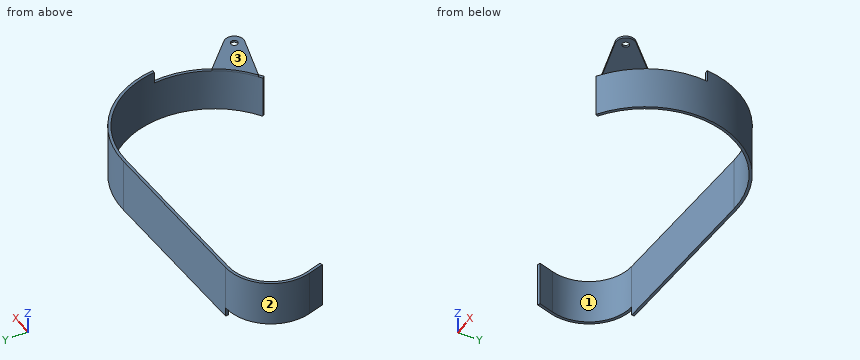
```python
from build123d import *

# Parameters (mm, degrees)
BASE_FLANGE1_DEPTH  = 52.5018
CUT_EXTRUDE1_DEPTH  = 8.89
CUT_EXTRUDE2_START  = -11.43
CUT_EXTRUDE2_DEPTH  = 11.43
SKETCH10_R          = 3.302
BOSS_EXTRUDE2_DEPTH = 2.032


# Sheet-metal steps are written as plain solids
with BuildPart() as part:
    # Sketch2 → Base-Flange1 (new body)
    with BuildSketch(Plane.XY):
        with BuildLine():
            Line((-203.2, 12.573), (-207.631458356, 27.163090613))
            ThreePointArc((-207.631458356, 27.163090613), (-201.190368302, 66.028990192), (-166.399327165, 84.512205491))
            Line((-166.399327165, 84.512205491), (-2.61152029, 89.301967603))
            ThreePointArc((-2.61152029, 89.301967603), (85.351357983, 26.397104888), (48.26, -75.184))
            Line((48.26, -75.184), (46.819332757, -72.939592084))
            ThreePointArc((46.819332757, -72.939592084), (82.803432048, 25.609093195), (-2.533560661, 86.636107274))
            Line((-2.533560661, 86.636107274), (-166.321367535, 81.846345161))
            ThreePointArc((-166.321367535, 81.846345161), (-199.024946204, 64.47212278), (-205.079570854, 27.938177176))
            Line((-205.079570854, 27.938177176), (-200.648112499, 13.348086563))
            Line((-200.648112499, 13.348086563), (-203.2, 12.573))
        make_face()
    extrude(amount=BASE_FLANGE1_DEPTH)

    # Sketch7 → Cut-Extrude1 (cut)
    with BuildSketch(Plane(origin=(0, 0, 0), x_dir=(-1, 0, 0), z_dir=(0, 0, -1))):
        with BuildLine():
            Line((166.399327165, 84.512205491), (166.321367535, 81.846345161))
            ThreePointArc((166.321367535, 81.846345161), (199.024946204, 64.47212278), (205.079570854, 27.938177176))
            Line((205.079570854, 27.938177176), (200.648112499, 13.348086563))
            Line((200.648112499, 13.348086563), (203.2, 12.573))
            Line((203.2, 12.573), (207.631458356, 27.163090613))
            ThreePointArc((207.631458356, 27.163090613), (201.190368302, 66.028990192), (166.399327165, 84.512205491))
        make_face()
    extrude(amount=-CUT_EXTRUDE1_DEPTH, mode=Mode.SUBTRACT)

    # Sketch9 → Cut-Extrude2 (cut)
    with BuildSketch(Plane.XY.offset(52.5018).offset(CUT_EXTRUDE2_START)):
        with BuildLine():
            Line((46.819332757, -72.939592084), (48.26, -75.184))
            ThreePointArc((48.26, -75.184), (80.427121635, -38.89909461), (88.901213224, 8.845097132))
            Line((88.901213224, 8.845097132), (86.220637146, 8.845097132))
            ThreePointArc((86.220637146, 8.845097132), (78.083879549, -37.618370083), (46.819332757, -72.939592084))
        make_face()
    extrude(amount=CUT_EXTRUDE2_DEPTH, mode=Mode.SUBTRACT)

    # Sketch10 → Boss-Extrude2 (add)
    with BuildSketch(Plane.XY.offset(41.0718)):
        with BuildLine():
            Line((76.378066867, -40.971025307), (103.240982904, -67.736900681))
            ThreePointArc((103.240982904, -67.736900681), (104.68136366, -78.663063475), (94.486544869, -82.848920608))
            Line((94.486544869, -82.848920608), (50.096351047, -70.728987162))
            ThreePointArc((50.096351047, -70.728987162), (64.964056756, -57.375128261), (76.378066867, -40.971025307))
        make_face()
        with Locations((96.865618573, -74.135379129)):
            Circle(SKETCH10_R, mode=Mode.SUBTRACT)
    extrude(amount=BOSS_EXTRUDE2_DEPTH)


solid = part.part
```
CAD build for the part. Positions are in the model's coordinates, mm. Face numbers are marked on the shaded views. Coordinates: 2 decimals unless noted, no trailing zeros. Write each loop counter-clockwise with the first axis right and the second up, starting at its lowest first coordinate (ties: lowest second). Pieces come first, ordered by that corner, then holes.
(1) Cut at C-C, the plane z = 28. List the corners of the cut face in (x, y), and give its area (3 significant figures).
(2) Cut at A-A, the plane y = 56. List the corners of the cut face in (x, z), and give its area (3 significant figures).
(3) Cut at D-D, the plane y = -59.5. List the corners of the cut face in (x, z), and give its area (3 significant figures).
(4) Flat gauge pins, fed straight in: pin 1 (21 mm diameter, centred on x = 90, y = -62, fed in from +Z); pin 2 (1.5 mm diameter, centred on y = 15, z = 36, fed in from +X); pin 3 (4 mm diameter, centred on x = 85, y = -24, fed in from +Z). Where does each tip first touch, or does it go through?
(5) Drill centre lines: probe 1 along Y at (x, z) = (-167.5, 49); probe 2 along Y at (x, z) = (-0.5, 41); probe 3 along X at (y, z) = (56, 30). Where is each one in solid material? Low to high.
(6) Two-plate mould, pull along X, no slides. Class the marked faces 1, 2 and 3: +X half, -X half, draft (parallel to the pull), parting line (faces both ways), or undercut.
(7) Cut at B-B, the plane x = 83. List the corners of the cut face in (y, z), and give its area (3 significant figures).
Geometry says:
1. outline: (-207.63, 27.16) - (-203.2, 12.57) - (-200.65, 13.35) - (-205.08, 27.94) arc R41.78 cw to (-166.32, 81.85) - (-2.53, 86.64) arc R86.67 cw to (46.82, -72.94) - (48.26, -75.18) arc R89.34 ccw to (-2.61, 89.3) - (-166.4, 84.51) arc R44.45 ccw to start
1. area: 1,300 mm2
2. outline: (-206.6, 8.89) - (-203.73, 8.89) - (-203.73, 52.5) - (-206.6, 52.5) - close; (66.15, 0) - (69.61, 0) - (69.61, 52.5) - (66.15, 52.5) - close
2. area: 307 mm2
3. outline: (63.02, 0) - (66.64, 0) - (66.64, 41.07) - (94.97, 41.07) - (94.97, 43.1) - (63.02, 43.1) - close
3. area: 214 mm2
4. pin 1: stops at z = 43.1
4. pin 2: stops at x = 88.2
4. pin 3: stops at z = 41.07
5. probe 1: y = 81.8 to 84.47
5. probe 2: y = 86.67 to 89.34
5. probe 3: x = -206.6 to -203.73, 66.15 to 69.61
6. face 1: undercut
6. face 2: -X half
6. face 3: draft
7. outline: (-79.71, 41.07) - (-47.57, 41.07) - (-47.57, 43.1) - (-79.71, 43.1) - close; (-33.06, 0) - (-24.96, 0) - (-24.96, 41.07) - (-33.06, 41.07) - close; (24.96, 0) - (33.06, 0) - (33.06, 52.5) - (24.96, 52.5) - close
7. area: 822 mm2
